```python
from build123d import *

# Parameters (mm, degrees)
BOSS_EXTRUDE2_DEPTH = 3
CUT_EXTRUDE2_DEPTH  = 5


with BuildPart() as part:
    # Sketch2 → Boss-Extrude2 (new body)
    with BuildSketch(Plane(origin=(0, 0, 0), x_dir=(1, 0, 0), z_dir=(0, 1, 0))):
        with BuildLine():
            Line((104.32233047, -139.67766953), (0, -35.355339059))
            Line((0, -35.355339059), (-104.32233047, -139.67766953))
            ThreePointArc((-104.32233047, -139.67766953), (-139.67766953, -139.67766953), (-139.67766953, -104.32233047))
            Line((-139.67766953, -104.32233047), (-35.355339059, 0))
            Line((-35.355339059, 0), (-139.67766953, 104.32233047))
            ThreePointArc((-139.67766953, 104.32233047), (-139.67766953, 139.67766953), (-104.32233047, 139.67766953))
            Line((-104.32233047, 139.67766953), (0, 35.355339059))
            Line((0, 35.355339059), (104.32233047, 139.67766953))
            ThreePointArc((104.32233047, 139.67766953), (139.67766953, 139.67766953), (139.67766953, 104.32233047))
            Line((139.67766953, 104.32233047), (35.355339059, 0))
            Line((35.355339059, 0), (139.67766953, -104.32233047))
            ThreePointArc((139.67766953, -104.32233047), (139.67766953, -139.67766953), (104.32233047, -139.67766953))
        make_face()
    extrude(amount=BOSS_EXTRUDE2_DEPTH)

    # Sketch6 → Cut-Extrude2 (cut)
    with BuildSketch(Plane(origin=(0, 3, 0), x_dir=(1, 0, 0), z_dir=(0, 1, 0))):
        Polygon((0, -14.142135624), (14.142135624, 0), (0, 14.142135624), (-14.142135624, 0), align=None)
    extrude(amount=-CUT_EXTRUDE2_DEPTH, mode=Mode.SUBTRACT)


solid = part.part
```
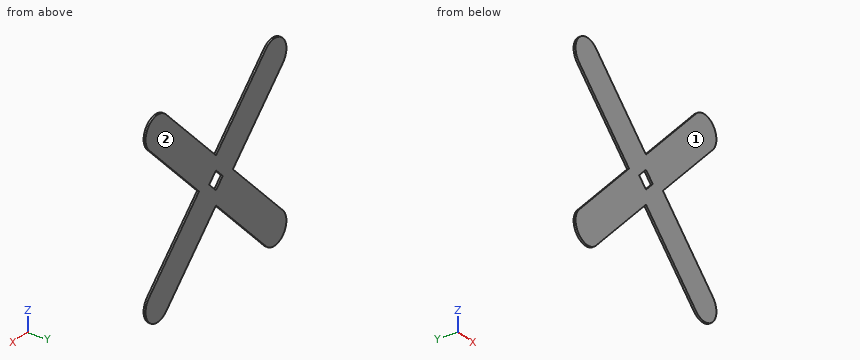
The model under review builds one solid part; all positions refer to its coordinate system, in mm. Face numbers are marked on the shaded views. Round coordinates to 2 decimals unless told otherwise and drop trailing zeros. Loops run counter-clockwise (first coordinate to the right, second up) from the corner with the lowest first, then second, coordinate; pieces in that order, holes last. Notation, with made-up numbers: (48, 24) - (73, 24) arc R20 cw to (73, 36) - close; hole circle Ø8 at (70, -26). An arc over 180 degrees is marked (long way). Use a Markdown table: item, result. Add a question column.
Q1. Insertion check: pin 1 Ø8 at (x, z) = (-64, 21.5) entering from +Y. The pin has a flat end and moves straight along its axis. Give the tip position at first contact, or say it passes through.
Q2. For probe 1 along X at (y, z) = (1.8, -129); probe 2 along X at (y, z) = (0.3, -60); probe 3 along Z at (x, y) = (89.5, 1.65), list the stretches that pass through material, from the lowest coordinate up.
Q3. Add section B-B (z = 122). State the section outline as (x, y) points.
Q4. Add section A-A (x = 73). State the section outline as (y, z) points.
Q5. The part is to be moulded in two halves that separate along Y. For the marked faces 1 and 2, say which applies: pulls with the +Y half, pulls with the -Y half, needs draft (parallel to the pull), parting line crosses it, or undercut.
Q6. Add section C-C (z = 32). State the section outline as (x, y) points, plus the area to 3 significant figures.
Q7. Add section D-D (x = 25). State the section outline as (y, z) points, plus the area to 3 significant figures.
Worked answers:
| question | item | result |
|---|---|---|
| 1 | pin 1 | through |
| 2 | probe 1 | -146 to -93.64, 93.64 to 146 |
| 2 | probe 2 | -95.36 to -24.64, 24.64 to 95.36 |
| 2 | probe 3 | -124.86 to -54.14, 54.14 to 124.86 |
| 3 | outline | (-147, 0) - (-86.64, 0) - (-86.64, 3) - (-147, 3) - close; (86.64, 0) - (147, 0) - (147, 3) - (86.64, 3) - close |
| 4 | outline | (0, -108.36) - (3, -108.36) - (3, -37.64) - (0, -37.64) - close; (0, 37.64) - (3, 37.64) - (3, 108.36) - (0, 108.36) - close |
| 5 | face 1 | pulls with the -Y half |
| 5 | face 2 | pulls with the +Y half |
| 6 | outline | (-67.36, 0) - (67.36, 0) - (67.36, 3) - (-67.36, 3) - close |
| 6 | area | 404 mm² |
| 7 | outline | (0, -60.36) - (3, -60.36) - (3, 60.36) - (0, 60.36) - close |
| 7 | area | 362 mm² |
